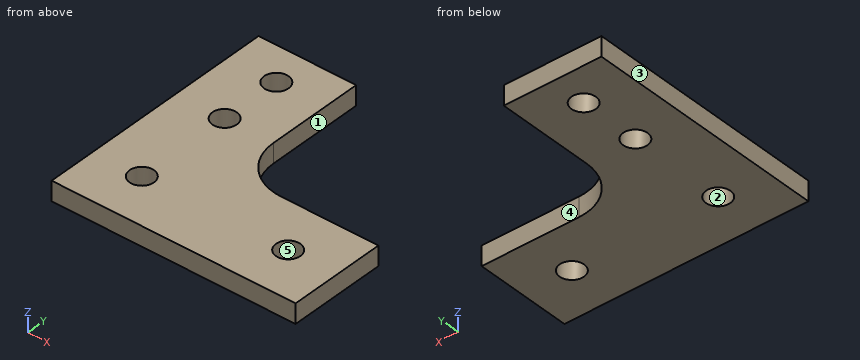
from build123d import *

# Parameters (mm, degrees)
SKETCH1_R           = 2.5
BOSS_EXTRUDE1_DEPTH = 4
FILLET1_R           = 10


with BuildPart() as part:
    # Sketch1 → Boss-Extrude1 (new body)
    with BuildSketch(Plane.XY):
        Polygon((-20, -10), (-20, 40), (0, 40), (0, 20), (0, 10), (10, 10), (30, 10), (30, -10), align=None)
        with Locations((-10, 32.5)):
            Circle(SKETCH1_R, mode=Mode.SUBTRACT)
        with Locations((-10, 0)):
            Circle(SKETCH1_R, mode=Mode.SUBTRACT)
        with Locations((20, 0)):
            Circle(SKETCH1_R, mode=Mode.SUBTRACT)
        with Locations((-10, 20)):
            Circle(SKETCH1_R, mode=Mode.SUBTRACT)
    extrude(amount=BOSS_EXTRUDE1_DEPTH)

    # Fillet1
    fillet1_edges = [part.edges().sort_by_distance(p)[0] for p in [
        (0, 10, 2),
    ]]
    fillet(fillet1_edges, radius=FILLET1_R)


solid = part.part
For this review, take the finished solid that the model builds, in its own axes (mm). Face numbers are marked on the shaded views. A direction names the side the tool comes from. Coordinates: 2 decimals unless noted, no trailing zeros. Write each loop counter-clockwise with the first axis right and the second up, starting at its lowest first coordinate (ties: lowest second). Pieces come first, ordered by that corner, then holes. Notation, with made-up numbers: (64, 25) -> (94, 25) arc R14 ccw to (94, 48) -> close; hole circle Ø4 at (9, -14.5). An arc over 180 degrees is marked (long way). Write each question's results on one line, items separated by ' | '. Start each with the question number.
1) Consider section B-B (x = 20). Write out the cut boundary in (y, z).
2) Consider section C-C (z = 1.9). Write out the cut boundary in (x, y), plus the area to 3 significant figures.
3) The part is to be moulded in two halves that separate along Y. For the marked faces 3, 4 and 5, say which applies: +Y half, -Y half, draft (parallel to the pull), parting line (faces both ways), or undercut.
4) For the marked faces 1 and 2, list the 3-axis set-ups (+Z, -Z, +X, -X, +Y, -Y) from which the entire face can be reached by the end or side of a thin tool; tool diameter is ignored.
5) Consider section A-A (y = 0). Write out the cut boundary in (x, z).
6) Consider section D-D (y = 21.5). Write out the cut boundary in (x, z), plus the area to 3 significant figures.
7) Insertion check: pin 1 (3 mm diameter, centred on x = -10, y = 32.5, fed in from +Z); pin 2 (1.2 mm diameter, centred on y = 33, z = 1.5, fed in from +X); pin 3 (1.5 mm diameter, centred on y = 16, z = 1.5, fed in from +X); pin 4 (2 mm diameter, centred on x = 20, z = 2, fed in from +Y). Each pin has a flat end and moves straight along its axis. Give the tip position at first contact, or say it passes through.
8) Wall thickness on L1, parallel to Y at x = -10, z = 2.5; L2, parallel to Y at x = 20, z = 1.7; L3, parallel to X at y = -1, z = 0.75: over which ranges is each line inside the solid? List them lowest first. Write a range as [from, to].
Geometry says:
1) outline: (-10, 0) -> (-2.5, 0) -> (-2.5, 4) -> (-10, 4) -> close; (2.5, 0) -> (10, 0) -> (10, 4) -> (2.5, 4) -> close
2) outline: (-20, -10) -> (30, -10) -> (30, 10) -> (10, 10) arc R10 cw to (0, 20) -> (0, 40) -> (-20, 40) -> close; hole circle Ø5 at (-10, 0); hole circle Ø5 at (-10, 20); hole circle Ø5 at (-10, 32.5); hole circle Ø5 at (20, 0) | area: 1,540 mm^2
3) face 3: draft | face 4: +Y half | face 5: undercut
4) face 1: +Z, -Z, +X, +Y | face 2: +Z, -Z
5) outline: (-20, 0) -> (-12.5, 0) -> (-12.5, 4) -> (-20, 4) -> close; (-7.5, 0) -> (17.5, 0) -> (17.5, 4) -> (-7.5, 4) -> close; (22.5, 0) -> (30, 0) -> (30, 4) -> (22.5, 4) -> close
6) outline: (-20, 0) -> (-12, 0) -> (-12, 4) -> (-20, 4) -> close; (-8, 0) -> (0, 0) -> (0, 4) -> (-8, 4) -> close | area: 64.0 mm^2
7) pin 1: through | pin 2: x = 0 | pin 3: x = 1.2 | pin 4: y = 10
8) L1: [-10, -2.5], [2.5, 17.5], [22.5, 30], [35, 40] | L2: [-10, -2.5], [2.5, 10] | L3: [-20, -12.29], [-7.71, 17.71], [22.29, 30]
